Can you work these out from the model? Positions are in its coordinate system, mm. Give positions to 0.01 mm unless a question says otherwise; leave off trailing zeros. Write each loop counter-clockwise with the first axis right and the second up, starting at its lowest first coordinate (ties: lowest second). Pieces come first, ordered by that corner, then holes.
```python
from build123d import *

# Parameters (mm, degrees)
F0_W     = 101.6
F0_H     = 25.4
F1_DEPTH = 228.6
F2_R     = 24.5364
F4_DEPTH = 25.4
F5_SIZE  = 20.32


with BuildPart() as f1:
    # F0 (on Right) → F1 (new body)
    with BuildSketch(Plane.YZ):
        with Locations((-50.8, 12.7)):
            Rectangle(F0_W, F0_H)
    extrude(amount=F1_DEPTH)

    # F2
    f2_edges = [f1.edges().sort_by_distance(p)[0] for p in [
        (114.3, 0, 25.4),
    ]]
    fillet(f2_edges, radius=F2_R)

    # F3 (on face) → F4 (cut)
    with BuildSketch(Plane(origin=(0, 0, 0), x_dir=(1, 0, 0), z_dir=(0, 0, -1))):
        Polygon((210.685179, 101.6), (228.6, 0), (228.6, 101.6), align=None)
    extrude(amount=-F4_DEPTH, mode=Mode.SUBTRACT)

    # F5
    f5_edges = [f1.edges().sort_by_distance(p)[0] for p in [
        (105.342589, -101.6, 25.4),
    ]]
    chamfer(f5_edges, length=F5_SIZE)

    # F6: F1 across plane


with BuildPart() as f1_1:
    add(f1.part)
    add(f1.part.mirror(Plane.YZ))


solid = f1_1.part
```
1) Suppose I cut it at B-B on z = 13. Write out the boundary of the cut face in (x, y).
Values follow:
outline: (-228.03, -3.21) - (-212.08, -93.68) - (212.08, -93.68) - (228.03, -3.21) - close
2) Suppose I cut it at C-C on y = -57. Write out the boundary of the cut face in (x, z).
Values follow:
outline: (-218.55, 0) - (218.55, 0) - (218.55, 25.4) - (-218.55, 25.4) - close
3) For pin 1 Ø12 at (y, z) = (-77.5, 21) entering from +X; pin 2 Ø3 at (x, z) = (96.5, 21.5) entering from +Y; pin 3 Ø12 at (x, z) = (133.5, 9.5) entering from +Y, each with a flat end and sliding along its axis, tell me the tip position at first contact or that it passes through.
Values follow:
pin 1: stops at x = 215.99
pin 2: stops at y = -9.18
pin 3: stops at y = -0.14
4) Suppose I cut it at A-A on x = -168. Write out the boundary of the cut face in (y, z).
Values follow:
outline: (-101.6, 0) - (0, 0) - (0, 0.86) arc R24.54 ccw to (-24.54, 25.4) - (-81.28, 25.4) - (-101.6, 5.08) - close
5) If we mould it in two halves opening along X, with no side actions, what happens to faces 1 (the face through (3, -91.58, 15.1)), 2 (the face through (-219.517, -51.511, 12.522)), 3 (the face through (219.517, -51.511, 12.522))? For each: +X half, -X half, draft (parallel to the pull), parting line (faces both ways), or undercut.
Values follow:
face 1: draft
face 2: -X half
face 3: +X half
6) Please list where these lines run through material, in increasing order: L1, parallel to X at y = -24, z = 4.25; L2, parallel to Y at x = 41.5, z = 9.5; L3, parallel to Z at x = 165, y = -82.5.
Values follow:
L1: x = -224.37 to 224.37
L2: y = -97.18 to -1.57
L3: z = 0 to 24.18
